```python
from build123d import *

# Parameters (mm, degrees)
F1_W      = 59.3920350075
F1_H      = 27.6011824608
F1_W_2    = 50.9779006243
F1_H_2    = 18.371000886
F2_DEPTH  = 25.4
F0_W      = 59.3920350075
F0_H      = 27.6011824608
F3_DEPTH  = 5.604719976
F18_DEPTH = 3.1209578738
F6_W      = 56.5673206002
F6_H      = 1.5604789369
F7_DEPTH  = 1.4987937175
F8_W      = 56.5673206002
F8_H      = 1.5604789369
F19_DEPTH = 1.4998847619
F5_W      = 21.3707275689
F5_H      = 1.5604789369
F9_DEPTH  = 1.382375136
F20_R     = 0.2935322564
F10_DEPTH = 0.3048
F21_R     = 0.254
F22_W     = 2.4601090699
F22_H     = 2.4032953017
F11_DEPTH = 2.1082
F12_R     = 0.5576398104
F13_DEPTH = 0.508
F14_R     = 0.50799
F23_W     = 2.4601090699
F23_H     = 2.4571502453
F15_DEPTH = 2.1082
F24_R     = 0.5965812211
F16_DEPTH = 0.508
F17_R     = 0.50799


# Not quite as in the source:
# - a fillet or chamfer is up to 0.001 mm smaller than in the source, because OpenCascade refuses the exact size


with BuildPart() as f2:
    # F1 (on face) → F2 (new body)
    with BuildSketch(Plane.XY):
        Rectangle(F1_W, F1_H)
        Rectangle(F1_W_2, F1_H_2, mode=Mode.SUBTRACT)
    extrude(amount=F2_DEPTH)

    # F0 (on Top) → F3 (join)
    with BuildSketch(Plane.XY):
        Rectangle(F0_W, F0_H)
    extrude(amount=-F3_DEPTH)

    # F4 (on face) → F18 (join)
    with BuildSketch(Plane.XY.offset(25.4)):
        Polygon((29.6960175037, -13.8005912304), (29.6960175037, -10.6853637844), (-26.8713030964, -10.6853637844), (-26.8713030964, 10.6853637844), (29.6960175037, 10.6853637844), (29.6960175037, 13.8005912304), (-29.6960175037, 13.8005912304), (-29.6960175037, -13.8005912304), align=None)
    extrude(amount=F18_DEPTH)

    # F6 (on face) → F7 (join)
    with BuildSketch(Plane.XZ.offset(-10.6853637844)):
        with Locations((1.4123572037, 27.7407184053)):
            Rectangle(F6_W, F6_H)
    extrude(amount=F7_DEPTH)

    # F8 (on face) → F19 (join)
    with BuildSketch(Plane(origin=(0, -10.6853637844, 0), x_dir=(-1, 0, 0), z_dir=(0, 1, 0))):
        with Locations((-1.4123572037, 27.7407184053)):
            Rectangle(F8_W, F8_H)
    extrude(amount=F19_DEPTH)

    # F5 (on face) → F9 (join)
    with BuildSketch(Plane.YZ.offset(-26.8713030964)):
        with Locations((0, 27.7407184053)):
            Rectangle(F5_W, F5_H)
    extrude(amount=F9_DEPTH)

    # F20 (on face) → F10 (join)
    with BuildSketch(Plane.XY.offset(25.4)):
        with Locations((25.8976798505, 0)):
            Circle(F20_R)
    extrude(amount=F10_DEPTH)

    # F21
    f21_edges = [f2.edges().sort_by_distance(p)[0] for p in [
        (25.604148, 0, 25.7048),
    ]]
    fillet(f21_edges, radius=F21_R)

    # F22 (on face) → F11 (join)
    with BuildSketch(Plane(origin=(0, 13.8005912304, 0), x_dir=(-1, 0, 0), z_dir=(0, 1, 0))):
        with Locations((0, 2.2958383197)):
            Rectangle(F22_W, F22_H)
    extrude(amount=F11_DEPTH)

    # F12 (on face) → F13 (join)
    with BuildSketch(Plane(origin=(0, 15.9087912304, 0), x_dir=(-1, 0, 0), z_dir=(0, 1, 0))):
        with Locations((0, 2.2958383197)):
            Circle(F12_R)
    extrude(amount=F13_DEPTH)

    # F14 (radius 0.508 in the source; OpenCascade refuses exactly that, so slightly less here)
    f14_edges = [f2.edges().sort_by_distance(p)[0] for p in [
        (0.55764, 16.416791, 2.295838),
    ]]
    fillet(f14_edges, radius=F14_R)

    # F23 (on face) → F15 (join)
    with BuildSketch(Plane.XZ.offset(13.8005912304)):
        with Locations((0, 2.3100455292)):
            Rectangle(F23_W, F23_H)
    extrude(amount=F15_DEPTH)

    # F24 (on face) → F16 (join)
    with BuildSketch(Plane.XZ.offset(15.9087912304)):
        with Locations((0, 2.3100455292)):
            Circle(F24_R)
    extrude(amount=F16_DEPTH)

    # F17 (radius 0.508 in the source; OpenCascade refuses exactly that, so slightly less here)
    f17_edges = [f2.edges().sort_by_distance(p)[0] for p in [
        (-0.596581, -16.416791, 2.310046),
    ]]
    fillet(f17_edges, radius=F17_R)


solid = f2.part
```
Source: CAD feature listing. Evaluate the final solid. Frame: model axes, mm. A direction names the side the tool comes from. Round coordinates to 2 decimals unless told otherwise and drop trailing zeros. Loops run counter-clockwise (first coordinate to the right, second up) from the corner with the lowest first, then second, coordinate; pieces in that order, holes last. Notation, with made-up numbers: M 48,50.25 L 87,50.25 A28 cw 87,85.25 Z; hole C -38,14.5 d3. An arc over 180 degrees is marked long. Use a Markdown table: item, result. Add a question column.
1. Mould query, pull axis Y, two halves, no side actions, for faces 1 (the flat face through (-25.489, 0, 13)), 2 (the flat face through (0, 15, 1.094)), 3 (the flat face through (1, 15.909, 2)). Classes: pulls with the +Y half, pulls with the -Y half, needs draft (parallel to the pull), parting line crosses it, or undercut.
2. Reachability of faces 4 (the flat face through (-2.6, 9.4, 26.96)), 5 (the flat face through (-1.23, 15, 2)), 6 (the flat face through (0, 15, 3.497)), 7 (the flat face through (25.489, 0, 13)), 8 (the flat face through (-25.489, 0, 28)) from +Z, -Z, +X, -X, +Y, -Y: full face, straight path, thin tool, end or side. Return the list, or none.
3. Section query C-C on x = -10. Return the cut outline in (y, z), then the cut area to 3 significant figures.
4. Section query B-B on y = -5. Return the cut outline in (x, z).
5. Line query: line 1 (Y direction, x = -22, z = 13); line 2 (X direction, y = -6, z = 11); line 3 (Z direction, x = -6, y = 7). Output: solid intervals per line, ascending.
6. Contact query for flat-ended pins moving along their axis: P1, Ø1.7, axis at y = -15, z = 2, coming from the -X side; P2, Ø1.7, axis at x = -0.5, y = 15, coming from the +Z side; P3, Ø9, axis at x = 3.5, y = 0, coming from the +Z side. Output: stop coordinate, or through.
7. Section query A-A on z = 6.5. Return the cut outline in (x, y), then the cut area to 3 significant figures.
Reported:
| question | item | result |
|---|---|---|
| 1 | face 1 | undercut |
| 1 | face 2 | needs draft |
| 1 | face 3 | pulls with the +Y half |
| 2 | face 4 | +X |
| 2 | face 5 | +Z, -Z, -X, +Y |
| 2 | face 6 | +Z, +X, -X, +Y |
| 2 | face 7 | +Z |
| 2 | face 8 | +Z, +X |
| 3 | outline | M -13.8,-5.6 L 13.8,-5.6 L 13.8,28.52 L 9.19,28.52 L 9.19,26.96 L 10.69,26.96 L 10.69,25.4 L 9.19,25.4 L 9.19,0 L -9.19,0 L -9.19,25.4 L -10.69,25.4 L -10.69,26.96 L -9.19,26.96 L -9.19,28.52 L -13.8,28.52 Z |
| 3 | area | 413 mm² |
| 4 | outline | M -29.7,-5.6 L 29.7,-5.6 L 29.7,25.4 L 25.49,25.4 L 25.49,0 L -25.49,0 L -25.49,25.4 L -26.87,25.4 L -26.87,26.96 L -25.49,26.96 L -25.49,28.52 L -29.7,28.52 Z |
| 5 | line 1 | y = -13.8 to -9.19, 9.19 to 13.8 |
| 5 | line 2 | x = -29.7 to -25.49, 25.49 to 29.7 |
| 5 | line 3 | z = -5.6 to 0 |
| 6 | P1 | stops at x = -1.23 |
| 6 | P2 | stops at z = 3.5 |
| 6 | P3 | stops at z = 0 |
| 7 | outline | M -29.7,-13.8 L 29.7,-13.8 L 29.7,13.8 L -29.7,13.8 Z; hole M -25.49,-9.19 L 25.49,-9.19 L 25.49,9.19 L -25.49,9.19 Z |
| 7 | area | 703 mm² |
